Read the model definition and answer for the solid it produces. Units are mm, in the model's axes. Face numbers are marked on the shaded views. A direction names the side the tool comes from. Give positions to 0.01 mm unless a question says otherwise; leave off trailing zeros. Write each loop counter-clockwise with the first axis right and the second up, starting at its lowest first coordinate (ties: lowest second). Pieces come first, ordered by that corner, then holes. Notation, with made-up numbers: (85, 67.5) -> (94, 67.5) arc R11 ccw to (94, 84.5) -> close; hole circle Ø11 at (-1, 13.5). An arc over 180 degrees is marked (long way). Use a Markdown table: item, result.
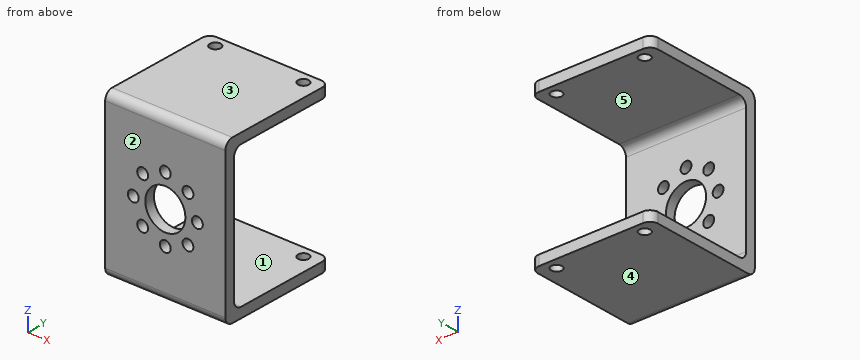
from build123d import *

# Parameters (mm, degrees)
ESBO_O1_W                = 30
ESBO_O1_H                = 30
RESSALTO_EXTRUS_O1_DEPTH = 40
ESBO_O2_W                = 35
ESBO_O2_H                = 27.5
CORTE_EXTRUS_O1_DEPTH    = 40
FILETE1_R                = 2
FILETE2_R                = 2
ESBO_O4_R                = 5
CORTE_EXTRUS_O3_DEPTH    = 53.201532545
ESBO_O5_R                = 1.35
CORTE_EXTRUS_O5_DEPTH    = 53.201532545
ESBO_O7_R                = 1.35
CORTE_EXTRUS_O6_DEPTH    = 46.276925691


with BuildPart() as part:
    # Esboço1 → Ressalto-extrusão1 (new body)
    with BuildSketch(Plane.XY):
        Rectangle(ESBO_O1_W, ESBO_O1_H)
    extrude(amount=RESSALTO_EXTRUS_O1_DEPTH)

    # Esboço2 → Corte-extrusão1 (cut)
    with BuildSketch(Plane(origin=(15, 0, 0), x_dir=(0, 0, -1), z_dir=(1, 0, 0))):
        with Locations((-20, 1.25)):
            Rectangle(ESBO_O2_W, ESBO_O2_H)
    extrude(amount=-CORTE_EXTRUS_O1_DEPTH, mode=Mode.SUBTRACT)

    # Filete1
    filete1_edges = [part.edges().sort_by_distance(p)[0] for p in [
        (-15, 15, 1.25),
        (15, 15, 1.25),
        (-15, 15, 38.75),
        (15, 15, 38.75),
    ]]
    fillet(filete1_edges, radius=FILETE1_R)

    # Filete2
    filete2_edges = [part.edges().sort_by_distance(p)[0] for p in [
        (0, -15, 40),
        (0, -12.5, 2.5),
        (0, -12.5, 37.5),
        (0, -15, 0),
    ]]
    fillet(filete2_edges, radius=FILETE2_R)

    # Esboço4 → Corte-extrusão3 (cut, through all)
    with BuildSketch(Plane(origin=(0, -15, 0), x_dir=(-1, 0, 0), z_dir=(0, -1, 0))):
        with Locations(Location((0, -20, 0), (0, 0, 90))):
            Circle(ESBO_O4_R)
    extrude(amount=-CORTE_EXTRUS_O3_DEPTH, mode=Mode.SUBTRACT)

    # Esboço5 → Corte-extrusão5 (cut, through all)
    with BuildSketch(Plane(origin=(0, -15, 0), x_dir=(-1, 0, 0), z_dir=(0, -1, 0))):
        with Locations(Location((0, -28, 0), (0, 0, 90))):
            Circle(ESBO_O5_R)
        with Locations(Location((-5.656854249, -25.656854249, 0), (0, 0, 90))):
            Circle(ESBO_O5_R)
        with Locations(Location((-8, -20, 0), (0, 0, 90))):
            Circle(ESBO_O5_R)
        with Locations(Location((-5.656854251, -14.343145752, 0), (0, 0, 90))):
            Circle(ESBO_O5_R)
        with Locations(Location((0, -12, 0), (0, 0, 90))):
            Circle(ESBO_O5_R)
        with Locations(Location((5.656854251, -14.343145752, 0), (0, 0, 90))):
            Circle(ESBO_O5_R)
        with Locations(Location((8, -20, 0), (0, 0, 90))):
            Circle(ESBO_O5_R)
        with Locations(Location((5.656854249, -25.656854249, 0), (0, 0, 90))):
            Circle(ESBO_O5_R)
    extrude(amount=-CORTE_EXTRUS_O5_DEPTH, mode=Mode.SUBTRACT)

    # Esboço7 → Corte-extrusão6 (cut, through all)
    with BuildSketch(Plane(origin=(0, 0, 0), x_dir=(-1, 0, 0), z_dir=(0, 0, -1))):
        with Locations((-11, 12.2)):
            Circle(ESBO_O7_R)
        with Locations((11, 12.2)):
            Circle(ESBO_O7_R)
    extrude(amount=-CORTE_EXTRUS_O6_DEPTH, mode=Mode.SUBTRACT)


solid = part.part
Item 1: For a pull along Z with two mould halves and no side action, classify the marked faces 3, 4 and 5 as +Z half, -Z half, draft (parallel to the pull), parting line (faces both ways), or undercut.
Return value:
| item | result |
|---|---|
| face 3 | +Z half |
| face 4 | -Z half |
| face 5 | undercut |
Item 2: A cutting plane is placed at D-D (y = 12.2). Give the vertices of the cut face in (x, z).
Return value:
| item | result |
|---|---|
| outline | (-15, 0) -> (-12.35, 0) -> (-12.35, 2.5) -> (-15, 2.5) -> close; (-15, 37.5) -> (-12.35, 37.5) -> (-12.35, 40) -> (-15, 40) -> close; (-9.65, 0) -> (9.65, 0) -> (9.65, 2.5) -> (-9.65, 2.5) -> close; (-9.65, 37.5) -> (9.65, 37.5) -> (9.65, 40) -> (-9.65, 40) -> close; (12.35, 0) -> (15, 0) -> (15, 2.5) -> (12.35, 2.5) -> close; (12.35, 37.5) -> (15, 37.5) -> (15, 40) -> (12.35, 40) -> close |
Item 3: Each of these flat-tipped pins is pushed along its axis until it touches: P1, Ø2, axis at x = -5.66, z = 14.34, coming from the -Y side; P2, Ø8, axis at x = -8.5, z = 26.5, coming from the +Y side. Where does it stop, or does it pass through?
Return value:
| item | result |
|---|---|
| P1 | through |
| P2 | y = -12.5 |
Item 4: A cutting plane is placed at A-A (y = 0.5). Give the vertices of the cut face in (x, z), then the cut area to 3 significant figures.
Return value:
| item | result |
|---|---|
| outline | (-15, 0) -> (15, 0) -> (15, 2.5) -> (-15, 2.5) -> close; (-15, 37.5) -> (15, 37.5) -> (15, 40) -> (-15, 40) -> close |
| area | 150 mm^2 |
Item 5: A cutting plane is placed at B-B (x = 11). Give the vertices of the cut face in (y, z), then the cut area to 3 significant figures.
Return value:
| item | result |
|---|---|
| outline | (-15, 2) arc R2 ccw to (-13, 0) -> (10.85, 0) -> (10.85, 2.5) -> (-10.5, 2.5) arc R2 cw to (-12.5, 4.5) -> (-12.5, 35.5) arc R2 cw to (-10.5, 37.5) -> (10.85, 37.5) -> (10.85, 40) -> (-13, 40) arc R2 ccw to (-15, 38) -> close; (13.55, 0) -> (15, 0) -> (15, 2.5) -> (13.55, 2.5) -> close; (13.55, 37.5) -> (15, 37.5) -> (15, 40) -> (13.55, 40) -> close |
| area | 224 mm^2 |
Item 6: A cutting plane is placed at C-C (z = 12). Give the vertices of the cut face in (x, y).
Return value:
| item | result |
|---|---|
| outline | (-15, -15) -> (-1.35, -15) -> (-1.35, -12.5) -> (-15, -12.5) -> close; (1.35, -15) -> (15, -15) -> (15, -12.5) -> (1.35, -12.5) -> close |
Item 7: Straight lines are drawn through the part: line 1 along X through (y, z) = (-13.55, 20); line 2 along Y through (x, z) = (-11, 38.1); line 3 along Z through (x, y) = (11, -9.5). For each, find the intervals that lie inside material, in ascending order. Write a range as [from, to].
Return value:
| item | result |
|---|---|
| line 1 | [-15, -9.35], [-6.65, -5], [5, 6.65], [9.35, 15] |
| line 2 | [-15, 10.85], [13.55, 15] |
| line 3 | [0, 2.5], [37.5, 40] |
Item 8: A tool of negligible diameter and unlimited length cuts with its end or side. For the marked faces 1 and 2, from which of +Z, -Z, +X, -X, +Y, -Y can it reach the whole face along a straight path? Write none if from no direction.
Return value:
| item | result |
|---|---|
| face 1 | +X, -X, +Y |
| face 2 | +Z, -Z, +X, -X, -Y |
